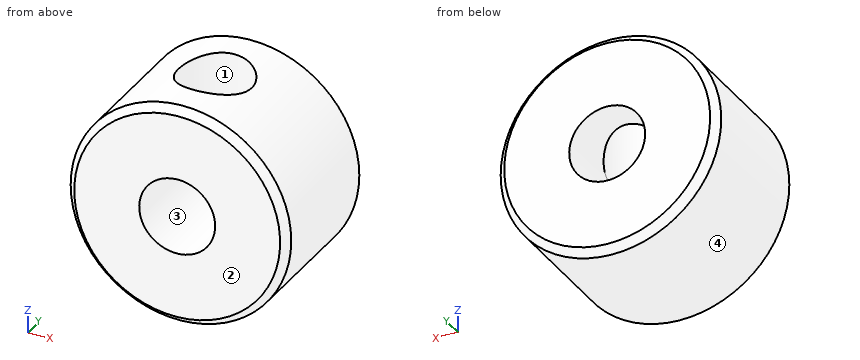
```python
from build123d import *

# Parameters (mm, degrees)
CROQUIS1_R                                     = 4.5
SALIENTE_EXTRUIR1_DEPTH                        = 6
CHAFL_N1_SIZE                                  = 0.3
CHAFL_N2_SIZE                                  = 0.3
CROQUIS2_R                                     = 1.55
CORTAR_EXTRUIR2_DEPTH                          = 6
PERFORADOR_PARA_ROSCAR_HELICOIL_DE_M2_21_REACH = 12.502
PERFORADOR_PARA_ROSCAR_HELICOIL_DE_M_2_R       = 1.5


with BuildPart() as part:
    # Croquis1 → Saliente-Extruir1 (new body)
    with BuildSketch(Plane(origin=(0, 0, 0), x_dir=(1, 0, 0), z_dir=(0, 1, 0))):
        with Locations(Location((0, 0, 0), (0, 0, 270))):
            Circle(CROQUIS1_R)
    extrude(amount=SALIENTE_EXTRUIR1_DEPTH)

    # Chaflán1
    chafl_n1_edges = [part.edges().sort_by_distance(p)[0] for p in [
        (0, 6, -4.5),
    ]]
    chamfer(chafl_n1_edges, length=CHAFL_N1_SIZE)

    # Chaflán2
    chafl_n2_edges = [part.edges().sort_by_distance(p)[0] for p in [
        (0, 0, -4.5),
    ]]
    chamfer(chafl_n2_edges, length=CHAFL_N2_SIZE)

    # Croquis2 → Cortar-Extruir2 (cut)
    with BuildSketch(Plane(origin=(0, 6, 0), x_dir=(1, 0, 0), z_dir=(0, 1, 0))):
        with Locations(Location((0, 0, 0), (0, 0, 270))):
            Circle(CROQUIS2_R)
    extrude(amount=-CORTAR_EXTRUIR2_DEPTH, mode=Mode.SUBTRACT)

    # Perforador para roscar Helicoil de M 2 (on position points) → Perforador para roscar Helicoil de M2.21 (cut, up to next)
    with BuildSketch(Plane(origin=(0.001317156, 3.003898977, 4.499999807), x_dir=(0.999999957163, 0, -0.000292701404), z_dir=(0.000292701404, 0, 0.999999957163)), mode=Mode.PRIVATE) as perforador_para_roscar_helicoil_de_m2_21_sk1:
        Circle(PERFORADOR_PARA_ROSCAR_HELICOIL_DE_M_2_R)
    perforador_para_roscar_helicoil_de_m2_21_tool1 = extrude(perforador_para_roscar_helicoil_de_m2_21_sk1.sketch, amount=-PERFORADOR_PARA_ROSCAR_HELICOIL_DE_M2_21_REACH, mode=Mode.PRIVATE) & part.part
    add(perforador_para_roscar_helicoil_de_m2_21_tool1.solids().sort_by_distance((0.001317, 3.003899, 4.5))[0], mode=Mode.SUBTRACT)


solid = part.part
```
Input: part model. Units: mm. Frame: model coordinates. Face numbers are marked on the shaded views. Coordinates: 2 decimals unless noted, no trailing zeros. Order: outer loops, then holes, each group sorted by start corner. A loop starts at its lowest first (then second) coordinate and runs counter-clockwise, first axis right, second up. Notation, with made-up numbers: (5, 22) - (63, 22) arc R10 ccw to (63, 26) - close; hole circle Ø1 at (70, 81.25). An arc over 180 degrees is marked (long way). Put each result on its own line as item: value.
1. Draft query along X for the marked faces 1, 2, 3 and 4. Return one class per face: pulls with the +X half, pulls with the -X half, needs draft (parallel to the pull), parting line crosses it, or undercut.
Report:
face 1: undercut
face 2: needs draft
face 3: undercut
face 4: parting line crosses it
2. Line query: line 1 along X through (y, z) = (3.5, 0); line 2 along Y through (x, z) = (-0.5, 4.25); line 3 along Y through (x, z) = (-0.5, 4). Output: solid intervals per line, ascending.
Report:
line 1: x = -4.5 to -1.55, 1.55 to 4.5
line 2: y = 0.08 to 1.59, 4.42 to 5.92
line 3: y = 0 to 1.59, 4.42 to 6
3. Cut plane A-A on z = 0. Return the cut outline in (x, y), then the cut area to 3 significant figures.
Report:
outline: (-4.5, 0.3) - (-4.2, 0) - (-1.55, 0) - (-1.55, 6) - (-4.2, 6) - (-4.5, 5.7) - close; (1.55, 0) - (4.2, 0) - (4.5, 0.3) - (4.5, 5.7) - (4.2, 6) - (1.55, 6) - close
area: 35.2 mm2
4. Cut plane D-D on y = 2.5. Return the cut outline in (x, z).
Report:
outline: (-1.41, 0.64) - (-1.41, 4.27) arc R4.5 ccw (long way) to (1.41, 4.27) - (1.41, 0.64) arc R1.55 cw (long way) to start
5. Cut plane C-C on x = 0. State how many separate pieces and enclosed holes the cut face has, then the cut area to 3 significant figures.
Report:
separate pieces: 3
enclosed holes: 0
area: 26.4 mm2
6. Cut plane B-B on y = 0.5. Return the cut outline in (x, z).
Report:
outline: circle Ø9 at (0, 0); hole circle Ø3.1 at (0, 0)
